from build123d import *

# Parameters (mm, degrees)
SKETCH1_R           = 1.6
BOSS_EXTRUDE1_DEPTH = 5
SKETCH2_R           = 2.5
BOSS_EXTRUDE2_DEPTH = 55
SKETCH5_W           = 8.290876423
SKETCH5_H           = 10
CUT_EXTRUDE1_DEPTH  = 0.5


with BuildPart() as part:
    # Sketch1 → Boss-Extrude1 (new body)
    with BuildSketch(Plane.XY):
        Circle(SKETCH1_R)
    extrude(amount=BOSS_EXTRUDE1_DEPTH)

    # Sketch2 → Boss-Extrude2 (add)
    with BuildSketch(Plane.XY.offset(5)):
        Circle(SKETCH2_R)
    extrude(amount=BOSS_EXTRUDE2_DEPTH)

    # Sketch4 → Groove for ANSI B27.7 - 3BM1-8, Basic Internal Retaining Ring1 (revolve, cut)
    with BuildSketch(Plane(origin=(0, 0, 54), x_dir=(0, 1, 0), z_dir=(-1, 0, 0)), mode=Mode.PRIVATE) as groove_for_ansi_b27_7_3bm1_8_basic_in_sk:
        with BuildLine():
            Line((4.1, -5), (2.14, -5))
            Line((2.14, -5), (2.14, -4.5))
            Line((2.14, -4.5), (4.1, -4.5))
            ThreePointArc((4.1, -4.5), (4.170710678, -4.529289322), (4.2, -4.6))
            Line((4.2, -4.6), (4.2, -4.9))
            ThreePointArc((4.2, -4.9), (4.170710678, -4.970710678), (4.1, -5))
        make_face()
    revolve(groove_for_ansi_b27_7_3bm1_8_basic_in_sk.sketch.rotate(Axis((0, -0.105559952, 104), (0, 0, -1)), 270), axis=Axis((0, -0.105559952, 104), (0, 0, -1)), mode=Mode.SUBTRACT)

    # Sketch5 → Cut-Extrude1 (cut)
    with BuildSketch(Plane.XZ.offset(2.5)):
        with Locations((-0.404897295, 15)):
            Rectangle(SKETCH5_W, SKETCH5_H)
    cut_extrude1 = extrude(amount=-CUT_EXTRUDE1_DEPTH, mode=Mode.SUBTRACT)

    # Mirror1: Cut-Extrude1 across plane
    add(cut_extrude1.mirror(Plane.ZX), mode=Mode.SUBTRACT)


solid = part.part
Geometry: final body of the model. Coordinates: model frame, mm. A direction names the side the tool comes from. Give positions to 0.01 mm unless a question says otherwise; leave off trailing zeros. Loops run counter-clockwise (first coordinate to the right, second up) from the corner with the lowest first, then second, coordinate; pieces in that order, holes last. Notation, with made-up numbers: (3.5, 72.25) - (29.5, 72.25) arc R10 cw to (29.5, 83.25) - close; hole circle Ø8 at (9, 65). An arc over 180 degrees is marked (long way). Answer as CSV lines item,"result". Start each with the question number.
1. Section A-A, the plane x = 0.35. Return loops of the section in (y, z), plus the area to 3 significant figures.
2. Section C-C, the plane y = -0.9. Return loops of the section in (x, z).
3. Section B-B, the plane z = 13.5. Return loops of the section in (x, y), plus the area to 3 significant figures.
4. Ray query, L1, parallel to Z at x = -2.05, y = 1.1; L2, parallel to X at y = 0.25, z = 25; L3, parallel to Z at x = 2, y = -0.9. Return the intervals inside material, ascending.
5. Reachability of faces 1 (the face through (1.782, -1.472, 58.746)), 2 (the face through (-1.27, -0.97, 2.46)), 3 (the face through (0, -2, 15)) from +Z, -Z, +X, -X, +Y, -Y: full face, straight path, thin tool, end or side. Return the list, or none.
6. Pin query (flat end, axial travel): P1, Ø2, axis at x = -1, z = 10.5, coming from the -Y side; P2, Ø2.5, axis at x = -0.5, z = 13.5, coming from the +Y side; P3, Ø1.5, axis at x = 0.5, z = 15.5, coming from the -Y side. Return the tip coordinate at first contact, or that it passes through.
7. Section D-D, the plane z = 38.5. Return loops of the section in (x, y), plus the area to 3 significant figures.
Answers:
1,outline,"(-2.48, 5) - (-1.56, 5) - (-1.56, 0) - (1.56, 0) - (1.56, 5) - (2.48, 5) - (2.48, 10) - (2, 10) - (2, 20) - (2.48, 20) - (2.48, 58.5) - (2.11, 58.5) - (2.11, 59) - (2.48, 59) - (2.48, 60) - (-2.48, 60) - (-2.48, 59) - (-2.32, 59) - (-2.32, 58.5) - (-2.48, 58.5) - (-2.48, 20) - (-2, 20) - (-2, 10) - (-2.48, 10) - close"
1,area,"278 mm2"
2,outline,"(-2.33, 5) - (-1.32, 5) - (-1.32, 0) - (1.32, 0) - (1.32, 5) - (2.33, 5) - (2.33, 58.5) - (2.1, 58.5) - (2.1, 59) - (2.33, 59) - (2.33, 60) - (-2.33, 60) - (-2.33, 59) - (-2.1, 59) - (-2.1, 58.5) - (-2.33, 58.5) - close"
3,outline,"(-1.5, -2) - (1.5, -2) arc R2.5 ccw to (1.5, 2) - (-1.5, 2) arc R2.5 ccw to start"
3,area,"17.6 mm2"
4,L1,"z = 5 to 58.5, 59 to 60"
4,L2,"x = -2.49 to 2.49"
4,L3,"z = 5 to 60"
5,face 1,"none"
5,face 2,"-Z"
5,face 3,"+X, -X, -Y"
6,P1,"stops at y = -2.5"
6,P2,"stops at y = 2"
6,P3,"stops at y = -2"
7,outline,"circle Ø5 at (0, 0)"
7,area,"19.6 mm2"
